from build123d import *

# Parameters (mm, degrees)
CROQUIS1_W              = 40
CROQUIS1_H              = 88
CROQUIS1_R              = 1.6
SALIENTE_EXTRUIR1_DEPTH = 15
CORTAR_EXTRUIR1_DEPTH   = 13
CROQUIS3_R              = 2.5
SALIENTE_EXTRUIR3_DEPTH = 2
CROQUIS4_R              = 1.25
CORTAR_EXTRUIR2_DEPTH   = 50.568134926
CROQUIS5_W              = 17.1
CROQUIS5_H              = 20.988594156
CROQUIS5_W_2            = 6.9
CORTAR_EXTRUIR3_DEPTH   = 51.606323716
SALIENTE_EXTRUIR4_START = -3
SALIENTE_EXTRUIR4_DEPTH = 3
CORTAR_EXTRUIR4_DEPTH   = 1
CROQUIS8_R              = 3
CORTAR_EXTRUIR5_DEPTH   = 51.606323716


with BuildPart() as part:
    # Croquis1 → Saliente-Extruir1 (new body)
    with BuildSketch(Plane(origin=(0, 0, 0), x_dir=(1, 0, 0), z_dir=(0, 1, 0))):
        Rectangle(CROQUIS1_W, CROQUIS1_H)
        with Locations(Location((-12, 40, 0), (0, 0, 270))):
            Circle(CROQUIS1_R, mode=Mode.SUBTRACT)
        with Locations(Location((12, 40, 0), (0, 0, 90))):
            Circle(CROQUIS1_R, mode=Mode.SUBTRACT)
        with Locations(Location((-12, -40, 0), (0, 0, 90))):
            Circle(CROQUIS1_R, mode=Mode.SUBTRACT)
        with Locations(Location((12, -40, 0), (0, 0, 270))):
            Circle(CROQUIS1_R, mode=Mode.SUBTRACT)
    extrude(amount=SALIENTE_EXTRUIR1_DEPTH)

    # Croquis2 → Cortar-Extruir1 (cut)
    with BuildSketch(Plane(origin=(0, 15, 0), x_dir=(1, 0, 0), z_dir=(0, 1, 0))):
        Polygon((-0.9, 48.396555715), (11.1, 48.396555715), (11.1, 16.5), (20, 16.5), (20, -37.5), (-20, -37.5), (-20, 16.5), (-0.9, 16.5), align=None)
    extrude(amount=-CORTAR_EXTRUIR1_DEPTH, mode=Mode.SUBTRACT)

    # Croquis3 → Saliente-Extruir3 (add)
    with BuildSketch(Plane(origin=(0, 2, 0), x_dir=(1, 0, 0), z_dir=(0, 1, 0))):
        with Locations(Location((11.1, 3, 0), (0, 0, 270))):
            Circle(CROQUIS3_R)
        with Locations(Location((4.1, -34.5, 0), (0, 0, 270))):
            Circle(CROQUIS3_R)
    extrude(amount=SALIENTE_EXTRUIR3_DEPTH)

    # Croquis4 → Cortar-Extruir2 (cut, through all)
    with BuildSketch(Plane(origin=(0, 4, 0), x_dir=(1, 0, 0), z_dir=(0, 1, 0))):
        with Locations(Location((11.1, 3, 0), (0, 0, 270))):
            Circle(CROQUIS4_R)
        with Locations(Location((4.1, -34.5, 0), (0, 0, 270))):
            Circle(CROQUIS4_R)
    extrude(amount=-CORTAR_EXTRUIR2_DEPTH, mode=Mode.SUBTRACT)

    # Croquis5 → Cortar-Extruir3 (cut, through all)
    with BuildSketch(Plane(origin=(0, 15, 0), x_dir=(1, 0, 0), z_dir=(0, 1, 0))):
        with Locations((-11.45, 26.994297078)):
            Rectangle(CROQUIS5_W, CROQUIS5_H)
        with Locations((16.55, 26.994297078)):
            Rectangle(CROQUIS5_W_2, CROQUIS5_H)
    extrude(amount=-CORTAR_EXTRUIR3_DEPTH, mode=Mode.SUBTRACT)

    # Croquis6 → Saliente-Extruir4 (add)
    with BuildSketch(Plane(origin=(0, 15, 0), x_dir=(1, 0, 0), z_dir=(0, 1, 0)).offset(SALIENTE_EXTRUIR4_START)):
        with BuildLine():
            Line((11.1, 44), (11.1, 41.322875656))
            ThreePointArc((11.1, 41.322875656), (10.4, 40), (11.1, 38.677124344))
            Line((11.1, 38.677124344), (11.1, 16.5))
            Line((11.1, 16.5), (-0.9, 16.5))
            Line((-0.9, 16.5), (-0.9, 44))
            Line((-0.9, 44), (11.1, 44))
        make_face()
    extrude(amount=SALIENTE_EXTRUIR4_DEPTH)

    # Croquis7 → Cortar-Extruir4 (cut)
    with BuildSketch(Plane(origin=(0, 0, -44), x_dir=(-1, 0, 0), z_dir=(0, 0, -1))):
        Polygon((-18.385000464, 9.353074792), (-13.054807804, 9.353074792), (-13.054807804, 8.645158579), (-13.596155496, 7.812315976), (-17.843652772, 7.812315976), (-18.385000464, 8.645158579), align=None)
    extrude(amount=-CORTAR_EXTRUIR4_DEPTH, mode=Mode.SUBTRACT)

    # Croquis8 → Cortar-Extruir5 (cut, through all)
    with BuildSketch(Plane.XZ):
        with Locations(Location((0, 25, 0), (0, 0, 270))):
            Circle(CROQUIS8_R)
        with Locations((0, -25)):
            Circle(CROQUIS8_R)
        with BuildLine():
            Line((-2.9, -16.5), (3.244083024, -1.312379042))
            ThreePointArc((3.244083024, -1.312379042), (1.312379042, 3.244083024), (-3.244083024, 1.312379042))
            Line((-3.244083024, 1.312379042), (-10.45, -16.5))
            Line((-10.45, -16.5), (-2.9, -16.5))
        make_face()
    extrude(amount=-CORTAR_EXTRUIR5_DEPTH, mode=Mode.SUBTRACT)


solid = part.part
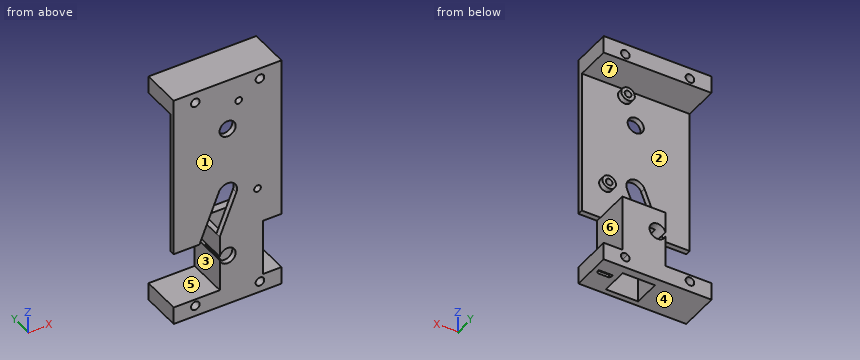
Verification items for the finished model (mm, model axes). Face numbers are marked on the shaded views. A direction names the side the tool comes from. Coordinates: 2 decimals unless noted, no trailing zeros. Loops run counter-clockwise (first coordinate to the right, second up) from the corner with the lowest first, then second, coordinate; pieces in that order, holes last. Notation, with made-up numbers: (37.25, -3.5) -> (75.25, -3.5) arc R19 ccw to (75.25, 21.5) -> close; hole circle Ø11 at (39, 20). An arc over 180 degrees is marked (long way). Answer as a JSON object with one key per item and string values. Group by question number.
Item 1: Sectioned sample at A-A on z = 34.5. Record the boundary of the cut face in (x, y), plus the area to 3 significant figures.
Item 2: Sectioned sample at D-D on z = -40. Record the boundary of the cut face in (x, y), plus the area to 3 significant figures.
Item 3: Scan lines: probe 1 along X at (y, z) = (9.75, 40); probe 2 along X at (y, z) = (6.75, -40); probe 3 along Z at (x, y) = (17.5, 8). Record each from-to range of solid material in increasing order.
Item 4: Mould release check, pull along Z, two halves, no side actions. Record for the marked faces 1, 2, 3 and 4: +Z half, -Z half, draft (parallel to the pull), parting line (faces both ways), or undercut.
Item 5: Sectioned sample at C-C on y = 6. Record the boundary of the cut face in (x, z).
Item 6: Tool access check on the marked faces 5, 6 and 7. Record the directions out of +Z, -Z, +X, -X, +Y, -Y that give a thin tool (end or side, any length) a straight path to the whole face; none if there is none.
Item 7: Sectioned sample at B-B on x = -12. Record the boundary of the cut face in (y, z), plus the area to 3 significant figures.
Item 8: Depth check by flat-ended pin: pin 1 (1.5 mm diameter, centred on x = 11, z = -2, fed in from +Y); pin 2 (6.5 mm diameter, centred on x = 6, y = 7.5, fed in from -Z); pin 3 (8 mm diameter, centred on y = 5, z = -33, fed in from +X). Enter the tip coordinate at first touch or a pass-through.
Evaluation:
{
 "1": {"outline": "(-20, 0) -> (2.85, 0) -> (2.85, 4) -> (1.6, 4) -> (1.6, 2) -> (-20, 2) -> close; (5.35, 0) -> (20, 0) -> (20, 2) -> (6.6, 2) -> (6.6, 4) -> (5.35, 4) -> close", "area": "80.0 mm²"},
 "2": {"outline": "(-20, 0) -> (-13.6, 0) -> (-13.6, 15) -> (-20, 15) -> close; (-10.4, 0) -> (10.4, 0) -> (10.4, 2) -> (-0.9, 2) -> (-0.9, 12) -> (10.4, 12) -> (10.4, 15) -> (-10.4, 15) -> close; (13.6, 0) -> (20, 0) -> (20, 15) -> (13.6, 15) -> close", "area": "391 mm²"},
 "3": {"probe 1": "x = -20 to -13.6, -10.4 to 10.4, 13.6 to 20", "probe 2": "x = -20 to -13.6, -10.4 to -0.9, 13.6 to 20", "probe 3": "z = -43 to -37.49, 37.5 to 44"},
 "4": {"face 1": "draft", "face 2": "undercut", "face 3": "undercut", "face 4": "-Z half"},
 "5": {"outline": "(-20, -44) -> (-0.9, -44) -> (-0.9, -27.86) arc R3 cw to (-2.9, -25.77) -> (-2.9, -37.49) -> (-20, -37.49) -> close; (-20, 37.5) -> (20, 37.5) -> (20, 44) -> (-20, 44) -> close; (-2.9, -24.23) arc R3 cw to (-0.9, -22.14) -> (-0.9, -16.5) -> (-2.9, -16.5) -> close; (11.1, -44) -> (20, -44) -> (20, -37.49) -> (13.1, -37.49) -> (13.1, -16.5) -> (11.1, -16.5) -> (11.1, -38.68) arc R1.6 cw (long way) to (11.1, -41.32) -> close; hole circle Ø3.2 at (-12, -40); hole circle Ø3.2 at (-12, 40); hole circle Ø3.2 at (12, 40)"},
 "6": {"face 5": "-X, +Y, -Y", "face 6": "+X, +Y, -Y", "face 7": "+X, -X, +Y"},
 "7": {"outline": "(0, -44) -> (15, -44) -> (15, -41.6) -> (0, -41.6) -> close; (0, -38.4) -> (15, -38.4) -> (15, -37.49) -> (0, -37.49) -> close; (0, -16.5) -> (2, -16.5) -> (2, 37.5) -> (15, 37.5) -> (15, 38.4) -> (0, 38.4) -> close; (0, 41.6) -> (15, 41.6) -> (15, 44) -> (0, 44) -> close", "area": "207 mm²"},
 "8": {"pin 1": "stops at y = 4", "pin 2": "stops at z = 37.5", "pin 3": "stops at x = 13.1"}
}
